from build123d import *

# Parameters (mm, degrees)
F0_W     = 177.8
F0_H     = 127
F1_DEPTH = 127
F2_T     = -25.4
F3_R     = 12.7


with BuildPart() as f1:
    # F0 (on Top) → F1 (new body)
    with BuildSketch(Plane.XY):
        with Locations((88.9, -63.5)):
            Rectangle(F0_W, F0_H)
    extrude(amount=F1_DEPTH)

    # F2
    f2_openings = [f1.faces().sort_by_distance(p)[0] for p in [
        (88.9, -63.5, 127),
    ]]
    offset(amount=F2_T, openings=f2_openings)

    # F3
    f3_edges = [f1.edges().sort_by_distance(p)[0] for p in [
        (152.4, -101.6, 76.2),
        (88.9, -101.6, 25.4),
        (25.4, -101.6, 76.2),
        (25.4, -25.4, 76.2),
        (25.4, -63.5, 25.4),
        (88.9, -25.4, 25.4),
        (152.4, -25.4, 76.2),
        (152.4, -63.5, 25.4),
        (177.8, 0, 63.5),
        (177.8, -127, 63.5),
        (0, -127, 63.5),
        (0, 0, 63.5),
    ]]
    fillet(f3_edges, radius=F3_R)


solid = f1.part
Could you check a few things on this model? Use its own coordinates, in mm. A direction names the side the tool comes from. Coordinates: 2 decimals unless noted, no trailing zeros. Write each loop counter-clockwise with the first axis right and the second up, starting at its lowest first coordinate (ties: lowest second). Pieces come first, ordered by that corner, then holes. Notation, with made-up numbers: M -13,4 L 13,4 A34 cw 13,40 Z; hole C 61,46.5 d1. An arc over 180 degrees is marked long. One line per question, with ' | ' between items.
1) Imagine slicing it at A-A, the plane y = -41.5. Write out the boundary of the cut face in (x, z).
Checks:
outline: M 0,0 L 177.8,0 L 177.8,127 L 152.4,127 L 152.4,38.1 A12.7 cw 139.7,25.4 L 38.1,25.4 A12.7 cw 25.4,38.1 L 25.4,127 L 0,127 Z
2) I need wall thicknesses on probe 1 along X at (y, z) = (-83.5, 37.5); probe 2 along Y at (x, z) = (78, 93.5); probe 3 along Z at (x, y) = (117, -54). Which ranges of each line are inside material? Lowest first, please. Write a range as [from, to].
Checks:
probe 1: [0, 25.41], [152.39, 177.8] | probe 2: [-127, -101.6], [-25.4, 0] | probe 3: [0, 25.4]
3) For pin 1 Ø12 at (x, y) = (84.5, -82.5) entering from +Z; pin 2 Ø5 at (x, y) = (46.5, -94.5) entering from +Z, each with a flat end and sliding along its axis, tell me the tip position at first contact or that it passes through.
Checks:
pin 1: z = 25.4 | pin 2: z = 28.32
4) For faces 1 (the face through (174.18, -3.82, 64.39)), 2 (the face through (88, -63, 25.4)), which set-ups out of +Z, -Z, +X, -X, +Y, -Y let a thin tool reach every point of the face, with its end or its side?
Checks:
face 1: +Z, -Z, +X, +Y | face 2: +Z
5) Imagine slicing it at C-C, the plane x = 126.5. Write out the boundary of the cut face in (y, z), and give its area (3 significant figures).
Checks:
outline: M -127,0 L 0,0 L 0,127 L -25.4,127 L -25.4,38.1 A12.7 cw -38.1,25.4 L -88.9,25.4 A12.7 cw -101.6,38.1 L -101.6,127 L -127,127 Z | area: 8,460 mm²
6) Imagine slicing it at B-B, the plane z = 64. Write out the boundary of the cut face in (x, y), and give its area (3 significant figures).
Checks:
outline: M 0,-114.3 A12.7 ccw 12.7,-127 L 165.1,-127 A12.7 ccw 177.8,-114.3 L 177.8,-12.7 A12.7 ccw 165.1,0 L 12.7,0 A12.7 ccw 0,-12.7 Z; hole M 25.4,-88.9 A12.7 ccw 38.1,-101.6 L 139.7,-101.6 A12.7 ccw 152.4,-88.9 L 152.4,-38.1 A12.7 ccw 139.7,-25.4 L 38.1,-25.4 A12.7 ccw 25.4,-38.1 Z | area: 12,900 mm²
7) If we mould it in two halves opening along X, with no side actions, what happens to faces 3 (the face through (25.4, -64, 82)), 4 (the face through (88, -20, 127)), 5 (the face through (3.62, -123.18, 64.39))? For each: released by +X, released by -X, zero draft, split by the parting line, or undercut.
Checks:
face 3: undercut | face 4: zero draft | face 5: released by -X
